Read the model definition and answer for the solid it produces. Units are mm, in the model's axes. A direction names the side the tool comes from. Coordinates: 2 decimals unless noted, no trailing zeros. Write each loop counter-clockwise with the first axis right and the second up, starting at its lowest first coordinate (ties: lowest second). Pieces come first, ordered by that corner, then holes.
(1) Section B-B on y = 47 is taken. Write down the section's boundary in (x, z).
(2) Given pin 1 (3 mm diameter, centred on y = 18.5, z = 8, fed in from +X); pin 2 (0.9 mm diameter, centred on x = 32.5, y = 40, fed in from +Z); pin 3 (9.5 mm diameter, centred on y = 62.31, z = 9.13, fed in from -X); pin 4 (5 mm diameter, centred on y = 62.31, z = 9.13, fed in from -X), each flat-ended and moving along its own axis, determine where each tip first touches the part or whether it passes through.
(3) Section C-C on x = 43 is taken. Write down the section's boundary in (y, z).
(4) Find the intervals of material crossed by probe 1 along X at (y, z) = (60.5, 14.75); probe 2 along Z at (x, y) = (16, 49); probe 3 along Y at (x, z) = (29.5, 14), in increasing order.
(5) Section A-A on z = 4.75 is taken. Write down the section's boundary in (x, y), then the cut area to 3 significant figures.
(6) Section D-D on z = 10.5 is taken. Write down the section's boundary in (x, y), then the cut area to 3 significant figures.
(7) Which of the six approach directions +Z, -Z, +X, -X, +Y, -Y give full straight-line access (tool end or side, diameter ignored) to faces 1 (the cylindrical face through (35.04, 2.85, 13.99)), 2 (the flat face through (14, 38, 2)), 3 (the flat face through (36.023, 37, 9)), 4 (the flat face through (30.977, 37, 9))?
(8) The mould has two halves that part along Z. Classify faces 5 (the flat face through (32, 38, 2)), 6 (the cylindrical face through (29.99, 65.08, 7.98)), 7 (the flat face through (32, 75, 1)), 8 (the cylindrical face through (35.037, 10.307, 7.308)): +Z half, -Z half, draft (parallel to the pull), parting line (faces both ways), or undercut.
from build123d import *

# Parameters (mm, degrees)
ESQUISSE1_W             = 65
ESQUISSE1_H             = 75
BOSS_EXTRU_1_DEPTH      = 2
ESQUISSE2_W             = 2
ESQUISSE2_H             = 75
BOSS_EXTRU_2_DEPTH      = 15
CONG_1_R                = 3
CONG_2_R                = 10
ESQUISSE6_R             = 3
ENL_V_MAT_EXTRU_1_DEPTH = 15


# Read off the part's stored shape, not the designer's step: Fraisage pour vis à tête fraisée M61
with BuildPart() as part:
    # Esquisse1 → Boss.-Extru.1 (new body)
    with BuildSketch(Plane.XY):
        with Locations((32.5, 37.5)):
            Rectangle(ESQUISSE1_W, ESQUISSE1_H)
    extrude(amount=BOSS_EXTRU_1_DEPTH)

    # Esquisse2 → Boss.-Extru.2 (add)
    with BuildSketch(Plane.XY.offset(2)):
        with Locations((29.976787497, 37.5)):
            Rectangle(ESQUISSE2_W, ESQUISSE2_H)
        with Locations((35.023212503, 37.5)):
            Rectangle(ESQUISSE2_W, ESQUISSE2_H)
    extrude(amount=BOSS_EXTRU_2_DEPTH)

    # Congé1
    cong_1_edges = [part.edges().sort_by_distance(p)[0] for p in [
        (0, 75, 1),
        (65, 75, 1),
        (65, 0, 1),
        (0, 0, 1),
    ]]
    fillet(cong_1_edges, radius=CONG_1_R)

    # Congé2
    cong_2_edges = [part.edges().sort_by_distance(p)[0] for p in [
        (35.023212503, 0, 17),
        (35.023212503, 75, 17),
        (29.976787497, 75, 17),
        (29.976787497, 0, 17),
    ]]
    fillet(cong_2_edges, radius=CONG_2_R)

    # Fraisage pour vis à tête fraisée M61 out → Fraisage pour vis à tête fraisée M61 (revolve, cut)
    with BuildSketch(Plane(origin=(50.511606252, 65, 0), x_dir=(1, 0, 0), z_dir=(0, -1, 0))):
        Polygon((6.3, 2), (0, 2), (0, 0), (4.3, 0), align=None)
    revolve(axis=Axis((50.511606252, 65, 0), (0, 0, 1)), mode=Mode.SUBTRACT)

    # Fraisage pour vis _ t_te frais_e M61 2 o → Fraisage pour vis _ t_te frais_e M61 2 (revolve, cut)
    with BuildSketch(Plane(origin=(50.511606252, 10, 0), x_dir=(1, 0, 0), z_dir=(0, -1, 0))):
        Polygon((6.3, 2), (0, 2), (0, 0), (4.3, 0), align=None)
    revolve(axis=Axis((50.511606252, 10, 0), (0, 0, 1)), mode=Mode.SUBTRACT)

    # Fraisage pour vis _ t_te frais_e M61 3 o → Fraisage pour vis _ t_te frais_e M61 3 (revolve, cut)
    with BuildSketch(Plane(origin=(14.488393748, 10, 0), x_dir=(1, 0, 0), z_dir=(0, -1, 0))):
        Polygon((6.3, 2), (0, 2), (0, 0), (4.3, 0), align=None)
    revolve(axis=Axis((14.488393748, 10, 0), (0, 0, 1)), mode=Mode.SUBTRACT)

    # Fraisage pour vis _ t_te frais_e M61 4 o → Fraisage pour vis _ t_te frais_e M61 4 (revolve, cut)
    with BuildSketch(Plane(origin=(14.488393748, 65, 0), x_dir=(1, 0, 0), z_dir=(0, -1, 0))):
        Polygon((6.3, 2), (0, 2), (0, 0), (4.3, 0), align=None)
    revolve(axis=Axis((14.488393748, 65, 0), (0, 0, 1)), mode=Mode.SUBTRACT)

    # Esquisse6 → Enlèv. mat.-Extru.1 (cut)
    with BuildSketch(Plane(origin=(36.023212503, 0, 0), x_dir=(0, 0, -1), z_dir=(1, 0, 0))):
        with Locations(Location((-9.133710771, 62.312214024, 0), (0, 0, 90))):
            Circle(ESQUISSE6_R)
        with Locations(Location((-9.133710771, 12.687785976, 0), (0, 0, 90))):
            Circle(ESQUISSE6_R)
    extrude(amount=-ENL_V_MAT_EXTRU_1_DEPTH, mode=Mode.SUBTRACT)


solid = part.part
Response:
1. outline: (0, 0) - (65, 0) - (65, 2) - (36.02, 2) - (36.02, 17) - (34.02, 17) - (34.02, 2) - (30.98, 2) - (30.98, 17) - (28.98, 17) - (28.98, 2) - (0, 2) - close
2. pin 1: stops at x = 36.02
2. pin 2: stops at z = 2
2. pin 3: stops at x = 28.98
2. pin 4: passes through
3. outline: (0, 0) - (75, 0) - (75, 2) - (0, 2) - close
4. probe 1: x = 28.98 to 30.98, 34.02 to 36.02
4. probe 2: z = 0 to 2
4. probe 3: y = 2.86 to 72.14
5. outline: (28.98, 0) - (30.98, 0) - (30.98, 75) - (28.98, 75) - close; (34.02, 0) - (36.02, 0) - (36.02, 75) - (34.02, 75) - close
5. area: 300 mm2
6. outline: (28.98, 0.63) - (30.98, 0.63) - (30.98, 10.02) - (28.98, 10.02) - close; (28.98, 15.36) - (30.98, 15.36) - (30.98, 59.64) - (28.98, 59.64) - close; (28.98, 64.98) - (30.98, 64.98) - (30.98, 74.37) - (28.98, 74.37) - close; (34.02, 0.63) - (36.02, 0.63) - (36.02, 10.02) - (34.02, 10.02) - close; (34.02, 15.36) - (36.02, 15.36) - (36.02, 59.64) - (34.02, 59.64) - close; (34.02, 64.98) - (36.02, 64.98) - (36.02, 74.37) - (34.02, 74.37) - close
6. area: 252 mm2
7. face 1: +Z, +X, -X, -Y
7. face 2: +Z, -X, +Y, -Y
7. face 3: +Z, +X, +Y, -Y
7. face 4: +Z, +Y, -Y
8. face 5: +Z half
8. face 6: undercut
8. face 7: draft
8. face 8: undercut
